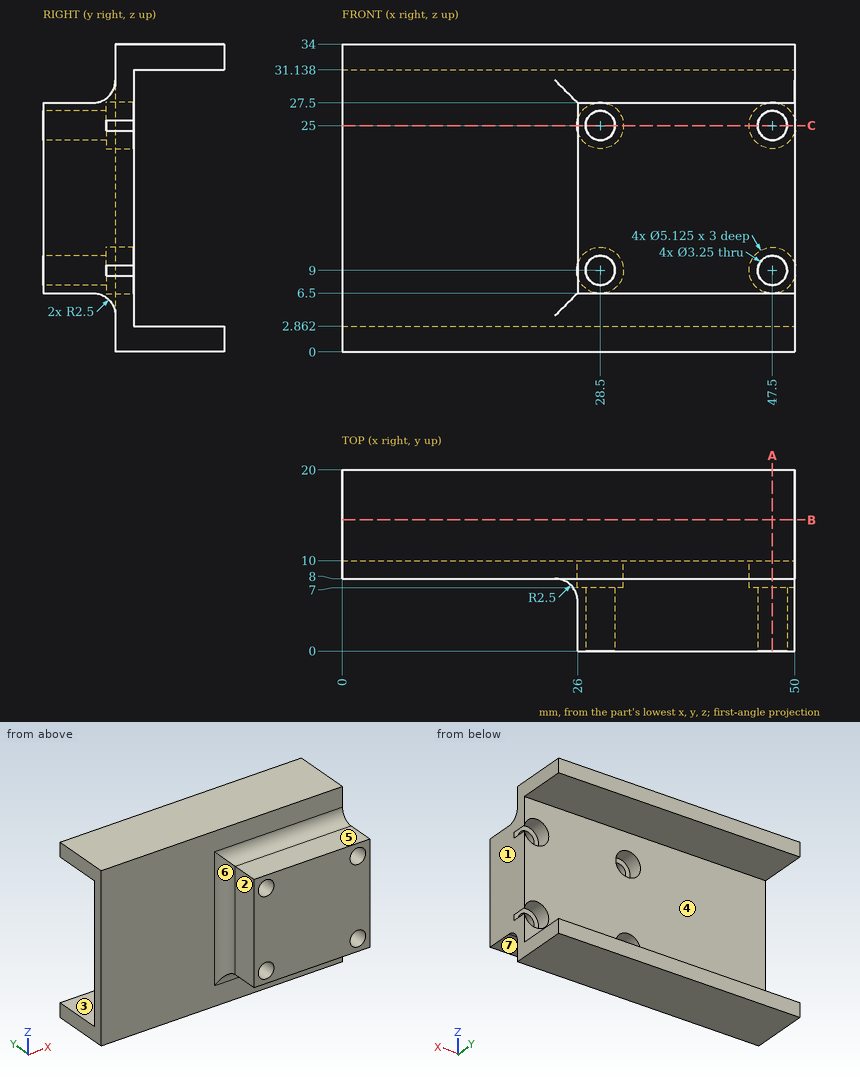
The drawing under review shows one solid part. Ordinate dimensions are in mm from its lowest x, y, z. A direction names the side the tool comes from. Coordinates: 2 decimals unless noted, no trailing zeros. Order: outer loops, then holes, each group sorted by start corner. A loop starts at its lowest first (then second) coordinate and runs counter-clockwise, first axis right, second up. Notation, with made-up numbers: M 36,2.25 L 59,2.25 A19 cw 59,35.25 Z; hole C 83.25,47 d6. An arc over 180 degrees is marked long. One line per question, with ' | ' between items.
(1) For probe 1 along X at (y, z) = (3.75, 25) (1 decimal); probe 2 along Z at (x, y) = (47.5, 9); probe 3 along Z at (x, y) = (47.5, 2.5) (1 decimal), list the stretches that pass through material, from the lowest coordinate up. Write a range as from..to.
Geometry results:
probe 1: x = 26..26.9, 30.1..45.9, 49.1..50 | probe 2: z = 0..6.44, 11.56..22.44, 27.56..34 | probe 3: z = 6.5..7.4, 10.6..23.4, 26.6..27.5
(2) Add section A-A, the plane x = 47.5. State how many separate pieces and enclosed holes the cut face has, then the cut area to 3 significant figures.
Geometry results:
separate pieces: 3 | enclosed holes: 0 | area: 220 mm²
(3) Add section C-C, the plane z = 25. Write out the cut boundary in (x, y) (1 decimal), then the cut area to 3 significant figures.
Geometry results:
outline: M 0,8 L 23.5,8 A2.5 cw 26,5.5 L 26,0 L 26.9,0 L 26.9,7 L 25.9,7 L 25.9,10 L 0,10 Z; M 30.1,0 L 45.9,0 L 45.9,7 L 44.9,7 L 44.9,10 L 31.1,10 L 31.1,7 L 30.1,7 Z; M 49.1,0 L 50,0 L 50,7 L 49.1,7 Z | area: 217 mm²
(4) The part is to be moulded in two halves that separate along Z. For the marked faces 4, 5, 6 and 7, say which applies: +Z half, -Z half, draft (parallel to the pull), parting line (faces both ways), or undercut.
Geometry results:
face 4: undercut | face 5: +Z half | face 6: draft | face 7: -Z half
(5) Insertion check: pin 1 (4.5 mm diameter, centred on x = 37, y = 2, fed in from -Z); pin 2 (4.5 mm diameter, centred on x = 40, y = 3, fed in from +Z); pin 3 (3 mm diameter, centred on x = 17, z = 24, fed in from -Y). Each pin has a flat end and moves straight along its axis. Give the tip position at first contact, or say it passes through.
Geometry results:
pin 1: stops at z = 6.5 | pin 2: stops at z = 27.5 | pin 3: stops at y = 8
(6) Add section B-B, the plane y = 14.5. Write out the cut boundary in (x, z).
Geometry results:
outline: M 0,0 L 50,0 L 50,2.86 L 0,2.86 Z; M 0,31.14 L 50,31.14 L 50,34 L 0,34 Z
(7) Machinability: for the marked faces 1, 2 and 3, which of the approach directions +Z, -Z, +X, -X, +Y, -Y give a long, thin tool a straight path to every point of the face, cutting with its end or side? Answer none if there is none.
Geometry results:
face 1: +Z, -Z, +X, +Y, -Y | face 2: +Z, -Z, -X, -Y | face 3: +X, -X, +Y
